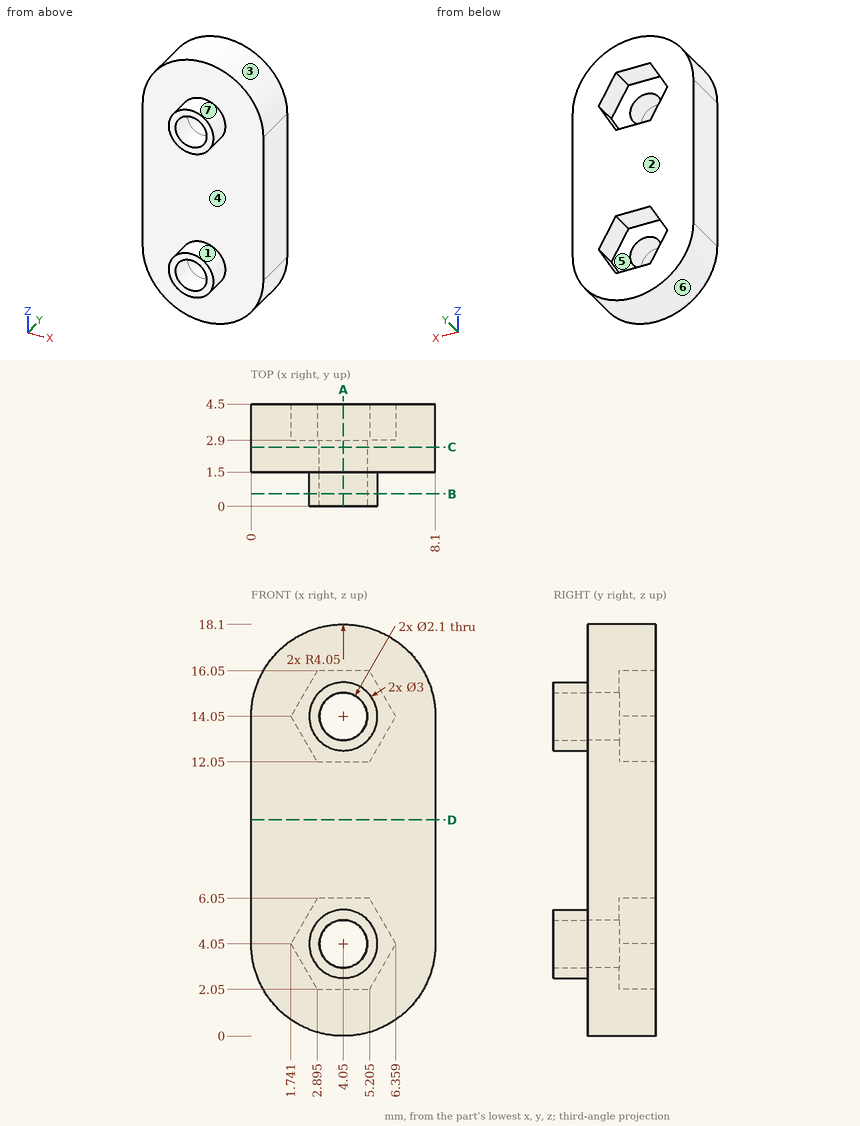
Input: dimensioned drawing with shaded views. Units: mm. Origin: part minimum x, y, z. A direction names the side the tool comes from. Coordinates: 2 decimals unless noted, no trailing zeros. Write each loop counter-clockwise with the first axis right and the second up, starting at its lowest first coordinate (ties: lowest second). Pieces come first, ordered by that corner, then holes. Notation, with made-up numbers: M 25.25,80 L 75.25,80 A6 cw 75.25,86 Z; hole C 38.5,38 d7. An arc over 180 degrees is marked long. Answer as a JSON object with one key per item and string values. Group by question number.
(1) Set-up query: the marked faces 5, 6 and 7. Return all of +Z, -Z, +X, -X, +Y, -Y with unobstructed straight access to the full face (end or side cutting, diameter ignored); none if empty.
(2) Section D-D on z = 9.5. Output: boundary loops of the cut face in (x, y), plus the area to 3 significant figures.
(3) Section A-A on x = 4.05. Output: boundary loops of the cut face in (y, z).
(4) Section B-B on y = 0.55. Output: boundary loops of the cut face in (x, z).
(5) Section C-C on y = 2.6. Output: boundary loops of the cut face in (x, z).
(6) Mould query, pull axis Z, two halves, no side actions, for the marked faces 1, 2, 3 and 4. Classes: pulls with the +Z half, pulls with the -Z half, needs draft (parallel to the pull), parting line crosses it, or undercut.
(7) Contact query for flat-ended pins moving along their axis: P1, Ø1.3, axis at x = 4.05, z = 14.05, coming from the -Y side; P2, Ø2.5, axis at x = 4.05, z = 4.05, coming from the -Y side; P3, Ø1.2, axis at x = 3, z = 14.5, coming from the +Y side; P4, Ø2, axis at x = 1, y = 3.5, coming from the -Z side. Output: stop coordinate, or through.
(8) Ray query, line 1 along Z through (x, y) = (4.05, 2.2); line 2 along Z through (x, y) = (4.05, 0.9); line 3 along Y through (x, z) = (5.5, 11). Return the intervals inside material, ascending. Write a range as [from, to].
Result set:
{
 "1": {"face 5": "+Y", "face 6": "-Z, +Y, -Y", "face 7": "-Y"},
 "2": {"outline": "M 0,1.5 L 8.1,1.5 L 8.1,4.5 L 0,4.5 Z", "area": "24.3 mm2"},
 "3": {"outline": "M 0,2.55 L 1.5,2.55 L 1.5,0 L 4.5,0 L 4.5,2.05 L 2.9,2.05 L 2.9,3 L 0,3 Z; M 0,5.1 L 2.9,5.1 L 2.9,6.05 L 4.5,6.05 L 4.5,12.05 L 2.9,12.05 L 2.9,13 L 0,13 L 0,12.55 L 1.5,12.55 L 1.5,5.55 L 0,5.55 Z; M 0,15.1 L 2.9,15.1 L 2.9,16.05 L 4.5,16.05 L 4.5,18.1 L 1.5,18.1 L 1.5,15.55 L 0,15.55 Z"},
 "4": {"outline": "C 4.05,4.05 d3; C 4.05,14.05 d3; hole C 4.05,4.05 d2.1; hole C 4.05,14.05 d2.1"},
 "5": {"outline": "M 0,4.05 A4.05 ccw 8.1,4.05 L 8.1,14.05 A4.05 ccw 0,14.05 Z; hole C 4.05,4.05 d2.1; hole C 4.05,14.05 d2.1"},
 "6": {"face 1": "undercut", "face 2": "needs draft", "face 3": "pulls with the +Z half", "face 4": "undercut"},
 "7": {"P1": "passes through", "P2": "stops at y = 0", "P3": "stops at y = 2.9", "P4": "stops at z = 0.56"},
 "8": {"line 1": "z = [0, 3], [5.1, 13], [15.1, 18.1]", "line 2": "z = [2.55, 3], [5.1, 5.55], [12.55, 13], [15.1, 15.55]", "line 3": "y = [1.5, 4.5]"}
}
